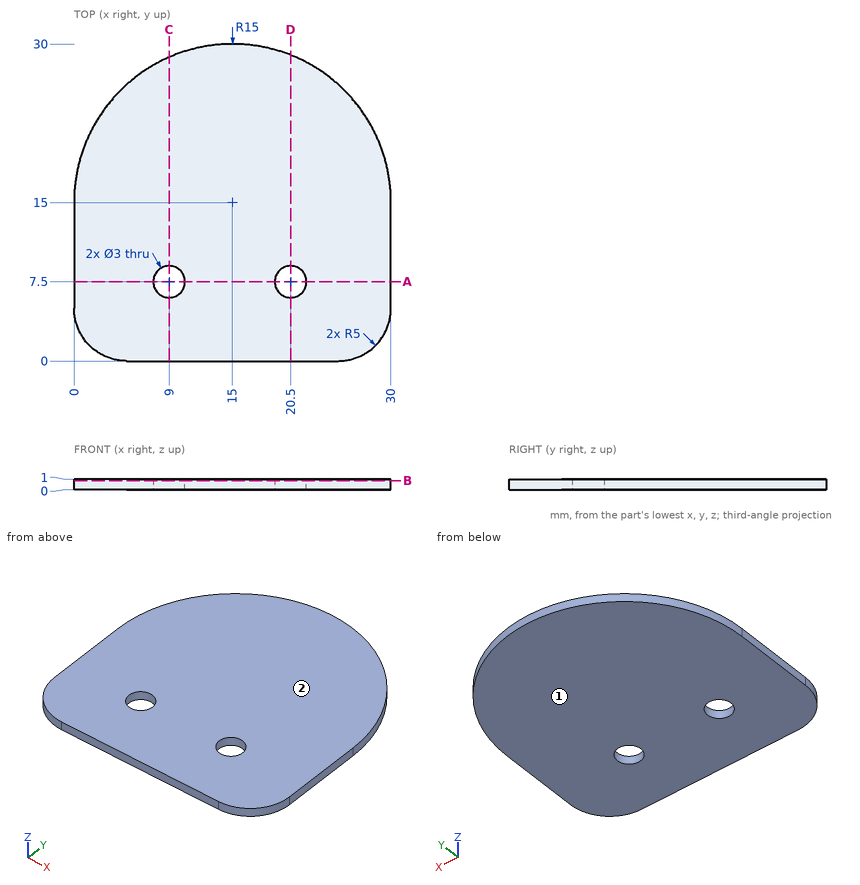
Verification items for this drawing (mm, ordinates from the low corner). Give positions to 0.01 mm unless a question says otherwise; leave off trailing zeros. Write each loop counter-clockwise with the first axis right and the second up, starting at its lowest first coordinate (ties: lowest second). Pieces come first, ordered by that corner, then holes.
1) Cross-section at B-B (z = 0.85). Record the boundary of the cut face in (x, y).
Values follow:
outline: (0, 5) arc R5 ccw to (5, 0) - (25, 0) arc R5 ccw to (30, 5) - (30, 15) arc R15 ccw to (0, 15) - close; hole circle Ø3 at (9, 7.5); hole circle Ø3 at (20.5, 7.5)
2) Release check for a two-part mould opening along Z. For the marked faces 1 and 2 record: released by +Z, released by -Z, zero draft, split by the parting line, or undercut.
Values follow:
face 1: released by -Z
face 2: released by +Z
3) Thickness scan on line 1 (X direction, y = 7, z = 0.7); line 2 (Y direction, x = 9, z = 0.45); line 3 (Y direction, x = 20.5, z = 0.4). Record the ranges inside material, lowest first.
Values follow:
line 1: x = 0 to 7.59, 10.41 to 19.09, 21.91 to 30
line 2: y = 0 to 6, 9 to 28.75
line 3: y = 0 to 6, 9 to 28.96
4) Cross-section at D-D (x = 20.5). Record the boundary of the cut face in (y, z), plus the area to 3 significant figures.
Values follow:
outline: (0, 0) - (6, 0) - (6, 1) - (0, 1) - close; (9, 0) - (28.96, 0) - (28.96, 1) - (9, 1) - close
area: 26.0 mm2
5) Cross-section at C-C (x = 9). Record the boundary of the cut face in (y, z), plus the area to 3 significant figures.
Values follow:
outline: (0, 0) - (6, 0) - (6, 1) - (0, 1) - close; (9, 0) - (28.75, 0) - (28.75, 1) - (9, 1) - close
area: 25.7 mm2
6) Cross-section at A-A (y = 7.5). Record the boundary of the cut face in (x, z).
Values follow:
outline: (0, 0) - (7.5, 0) - (7.5, 1) - (0, 1) - close; (10.5, 0) - (19, 0) - (19, 1) - (10.5, 1) - close; (22, 0) - (30, 0) - (30, 1) - (22, 1) - close
